Can you work these out from the model? Positions are in its coordinate system, mm. Coordinates: 2 decimals unless noted, no trailing zeros. Order: outer loops, then holes, each group sorted by start corner. A loop starts at its lowest first (then second) coordinate and runs counter-clockwise, first axis right, second up. Notation, with made-up numbers: (5.5, 7.25) - (28.5, 7.25) arc R23 ccw to (28.5, 33.25) - close; hole circle Ø10 at (17.5, -22). An arc over 180 degrees is marked (long way). Use a Markdown table: item, result. Add a question column.
(1) If I drill on L1, parallel to Y at x = 7.25, z = 0; L2, parallel to Z at x = 11, y = 1.25; L3, parallel to Y at x = 4, z = 0.75, over which ranges is the centre line in solid material (lowest first)? Write a range as [from, to].
(2) For pin 1 Ø4 at (x, z) = (34, 2) entering from +Y; pin 2 Ø4.5 at (y, z) = (0, 0) entering from -X; pin 3 Ø1 at (x, y) = (30, 2) entering from -Z; pin 4 Ø4 at (x, z) = (29, 4.5) entering from -Y, each with a flat end and sliding along its axis, tell me the tip position at first contact or that it passes through.
(3) I want a section at A-A (x = 6). List the corners of the cut face in (y, z) for me.
(4) I want a section at B-B (x = 33.5). List the corners of the cut face in (y, z) for me, and give its area (3 significant figures).
(5) We'd pull the mould along Z, two halves only. Please class faces 1 (the cylindrical face through (19.142, -1.802, 5.723)), 2 (the flat face through (40, 0, 0)), 3 (the conical face through (16.241, -0.424, -0.094)), 4 (the cylindrical face through (7.86, -2.44, 0.54)): pulls with the +Z half, pulls with the -Z half, needs draft (parallel to the pull), parting line crosses it, or undercut.
```python
from build123d import *

# Parameters (mm, degrees)
M6_GEWINDEBOHRUNG1_D           = 5
M6_GEWINDEBOHRUNG1_DEPTH       = 15
M6_GEWINDEBOHRUNG1_CSINK_D     = 6.05
M6_GEWINDEBOHRUNG1_CSINK_ANGLE = 90
M6_GEWINDEBOHRUNG1_TIP         = 1.502151548


with BuildPart() as part:
    # Skizze1 → Rotation3 (revolve)
    with BuildSketch(Plane.XY, mode=Mode.PRIVATE) as rotation3_sk:
        Polygon((0, 0), (0, 5.571281292), (1.6, 6), (36.2, 6), (40, 4.981793069), (40, 0), align=None)
    revolve(rotation3_sk.sketch.rotate(Axis((0, 0, 0), (1, 0, 0)), 90), axis=Axis((0, 0, 0), (1, 0, 0)))

    # M6 Gewindebohrung1
    with Locations(Plane.ZY):
        with Locations((0, 0)):
            CounterSinkHole(M6_GEWINDEBOHRUNG1_D / 2, M6_GEWINDEBOHRUNG1_CSINK_D / 2, depth=M6_GEWINDEBOHRUNG1_DEPTH, counter_sink_angle=M6_GEWINDEBOHRUNG1_CSINK_ANGLE)
            with Locations((0, 0, -(M6_GEWINDEBOHRUNG1_DEPTH + M6_GEWINDEBOHRUNG1_TIP / 2))):  # 118° drill point
                Cone(0, M6_GEWINDEBOHRUNG1_D / 2, M6_GEWINDEBOHRUNG1_TIP, mode=Mode.SUBTRACT)


solid = part.part
```
Answers follow:
| question | item | result |
|---|---|---|
| 1 | L1 | y = [-6, -2.5], [2.5, 6] |
| 1 | L2 | z = [-5.87, -2.17], [2.17, 5.87] |
| 1 | L3 | y = [-5.95, -2.38], [2.38, 5.95] |
| 2 | pin 1 | stops at y = 6 |
| 2 | pin 2 | stops at x = 15.15 |
| 2 | pin 3 | stops at z = -5.81 |
| 2 | pin 4 | stops at y = -5.45 |
| 3 | outline | circle Ø12 at (0, 0); hole circle Ø5 at (0, 0) |
| 4 | outline | circle Ø12 at (0, 0) |
| 4 | area | 113 mm² |
| 5 | face 1 | parting line crosses it |
| 5 | face 2 | needs draft |
| 5 | face 3 | undercut |
| 5 | face 4 | undercut |
